The listing builds one solid part. Answer for the finished solid, in the listing's coordinates (mm). A direction names the side the tool comes from. Coordinates: 2 decimals unless noted, no trailing zeros. Loops run counter-clockwise (first coordinate to the right, second up) from the corner with the lowest first, then second, coordinate; pieces in that order, holes last. Notation, with made-up numbers: (85, 23.25) - (101, 23.25) arc R31 cw to (101, 59.25) - close; hole circle Ø7 at (-3.5, 49). An arc over 180 degrees is marked (long way). One line per question, with ' | ' between items.
Autodesk Inventor part; units mm, degrees
ref_plane "Work Plane1" through (3.5, 0, 0) normal (0, 0, 1) x (1, 0, 0)
ref_plane "YZ Plane" through (0, 0, 0) normal (1, 0, 0) x (0, 1, 0)
ref_plane "XZ Plane" through (0, 0, 0) normal (0, 1, 0) x (-1, 0, 0)
sketch "Sketch1" plane through (0, 0, 0) normal (0, 0, 1) x (1, 0, 0)
  line L0 (0, 3.375) -> (0, 1.1933)
  line L1 (1, 1.5) -> (6, 1.5)
  line L2 (6, 1.5) -> (6, 0)
  line L3 (6, 0) -> (-0.53, 0)
  line L4 (0, -0.675) -> (0, 4.05)
  line L5 (-1.836, 0) -> (7.306, 0)
  line L6 (-0.53, 0) -> (-0.53, 3.375)
  line L7 (-0.53, 3.375) -> (0, 3.375)
  line L8 (1, 1.5) -> (0.6933, 1.1933)
  line L9 (0.6933, 1.1933) -> (0, 1.1933)
  dimension "d0" = 6
  dimension "d1" = 5
  dimension "d2" = 3
  dimension "d8" = 0.53
  dimension "d9" = 6.75
  dimension "d15" = 2.3866
  dimension "d16" = 0.3067
revolve "Body" add sketch "Sketch1" angle 360 about axis through (6, 0, 0) along (-1, 0, 0)
sketch "Sketch2" plane through (0, 0, 0) normal (1, 0, 0) x (0, 0, -1)
  circle A0 centre (0, 0) radius 3.375
  line L0 (0, 2.8868) -> (2.5, 1.4434)
  line L1 (2.5, 1.4434) -> (2.5, -1.4434)
  line L2 (2.5, -1.4434) -> (0, -2.8868)
  line L3 (0, -2.8868) -> (-2.5, -1.4434)
  line L4 (-2.5, -1.4434) -> (-2.5, 1.4434)
  line L5 (-2.5, 1.4434) -> (0, 2.8868)
  circle A1 centre (0, 0) radius 3.375
  dimension "d10" = 5
extrude "Head" add sketch "Sketch2" against normal blind 2.36 contours L0 L1 L2 L3 L4 L5
sketch "Sketch3" plane through (0, 0, 0) normal (0, 0, 1) x (1, 0, 0)
  line L0 (-2.36, 2.25) -> (-2.36, 2.8868)
  line L1 (-2.36, 2.8868) -> (-1.9924, 2.8868)
  line L2 (-1.9924, 2.8868) -> (-2.36, 2.25)
  line L3 (-1.7645, 2.8868) -> (-2.36, 2.8868)
  line L4 (-2.36, 2.8868) -> (-2.36, 0.5774)
  line L5 (-0.53, 2.8868) -> (-2.36, 2.8868)
  line L6 (-2.36, 2.8868) -> (-2.36, 1.4434)
  line L7 (-2.726, 0) -> (-0.164, 0)
  dimension "d5" = 30
  dimension "d18" = 4.5
revolve "Chamfer1" cut sketch "Sketch3" angle 360 about axis through (-10, 0, 0) along (1, 0, 0)
thread "Thread"
chamfer "Chamfer2" distance 0.3067 distance2 0.3068 1 edges at (6, -1.5, 0) measured on face at (6, -0.6587, 0.1791)
ref_plane "Work Plane1" through (3.5, 0, 0) normal (0, 0, 1) x (1, 0, 0)
equation "\"d0\" = NLG"
equation "\"d1\" = GEL"
equation "\"d2\" = GD"
equation "\"d8\" = PHH"
equation "\"d9\" = LADI"
equation "\"d15\" = BDM"
equation "\"d16\" = GAL"
equation "\"d10\" = SW"
equation "\"d3\" = KOH"
equation "\"d13\" = GEL"
equation "\"d6\" = -0.5 * SPD + 0.5 * GD"
equation "\"d5\" = ANG1"
equation "\"d18\" = SW0"
equation "\"NLG\" = 6"
equation "\"GD\" = NND"
equation "\"BDM\" = NND - 1.2269 * PTC"
equation "\"KOH\" = 2.36"
equation "\"GEL\" = 5"
equation "\"LADI\" = 6.75"
equation "\"SW\" = 5"
equation "\"PHH\" = 0.53"
equation "\"SW0\" = 4.5"
equation "\"SPD\" = NND - 1.2269 * PTC"
equation "\"ANG1\" = 30deg"
equation "\"GAL\" = 0.61345 * PTC"
equation "\"GUL\" = 0.61345 * PTC"
equation "\"WFT\" = PHH"
equation "\"PTC\" = 0.5"
equation "\"THREADDIA\" = 3"
equation "\"E0\" = 1.155 * SW"
equation "\"TOA\" = 30deg"
equation "\"NND\" = 3"
equation "\"GD1\" = THREADDIA - 1.2269 * PTC"
equation "\"SDH\" = 3.6"
equation "\"KOH1\" = 1.83"
equation "\"SD2\" = NND"
equation "\"SD\" = 0"
equation "\"RR\" = 0.1"
properties part number "AS 1427 - M3 X 6" material "Steel, High Strength Low Alloy"
Item 1: Find section D-D, the plane x = 4.5. Write down the section's boundary in (y, z).
Taken from the geometry:
outline: circle Ø3 at (0, 0)
Item 2: Each of these flat-tipped pins is pushed along its axis until it touches: pin 1 Ø4 at (x, y) = (3, 2.5) entering from -Z; pin 2 Ø0.8 at (x, y) = (-1, 0.5) entering from -Z. Where does it stop, or does it pass through?
Taken from the geometry:
pin 1: stops at z = -1.41 | pin 2: stops at z = -2.5
Item 3: Find the intervals of material crossed by line 1 (X direction, y = 3, z = 1); line 2 (X direction, y = 0.25, z = 1.25); line 3 (Z direction, x = 1.25, y = 0), in increasing order. Write a range as [from, to].
Taken from the geometry:
line 1: x = [-0.53, 0] | line 2: x = [-2.36, 0], [0.77, 5.92] | line 3: z = [-1.5, 1.5]
Item 4: Find section C-C, the plane z = 2.75. Write down the section's boundary in (x, y), plus the area to 3 significant figures.
Taken from the geometry:
outline: (-0.53, -1.96) - (0, -1.96) - (0, 1.96) - (-0.53, 1.96) - close | area: 2.07 mm2
Item 5: Find section A-A, the plane y = 0. Write down the section's boundary in (x, z) (3 decimals), plus the area to 3 significant figures.
Taken from the geometry:
outline: (-2.36, -2.25) - (-2.216, -2.5) - (-0.53, -2.5) - (-0.53, -3.375) - (0, -3.375) - (0, -1.193) - (0.693, -1.193) - (1, -1.5) - (5.693, -1.5) - (6, -1.193) - (6, 1.193) - (5.693, 1.5) - (1, 1.5) - (0.693, 1.193) - (0, 1.193) - (0, 3.375) - (-0.53, 3.375) - (-0.53, 2.5) - (-2.216, 2.5) - (-2.36, 2.25) - close | area: 30.1 mm2
Item 6: Find section B-B, the plane x = 0.5. Write down the section's boundary in (y, z).
Taken from the geometry:
outline: circle Ø2.39 at (0, 0)
Item 7: The mould has two halves that part along Z. Classify faces 4 (the face through (-1, 0, 2.5)), 5 (the face through (0.342, -0.88, -0.806)), 6 (the face through (-1.361, -2.155, -1.267)): pulls with the +Z half, pulls with the -Z half, needs draft (parallel to the pull), parting line crosses it, or undercut.
Taken from the geometry:
face 4: pulls with the +Z half | face 5: parting line crosses it | face 6: pulls with the -Z half
Item 8: Which of the six approach directions +Z, -Z, +X, -X, +Y, -Y give full straight-line access (tool end or side, diameter ignored) to faces 1 (the face through (-1.361, 2.155, 1.267)), 2 (the face through (-1, 0, -2.5)), 3 (the face through (-0.53, -1, -3))?
Taken from the geometry:
face 1: +Z, -X, +Y | face 2: -Z, -X, +Y, -Y | face 3: -X
